Work out the finished part from the listing and answer in its coordinate system (mm). A direction names the side the tool comes from. Round coordinates to 2 decimals unless told otherwise and drop trailing zeros. Write each loop counter-clockwise with the first axis right and the second up, starting at its lowest first coordinate (ties: lowest second). Pieces come first, ordered by that corner, then holes. Notation, with made-up numbers: (3, 21.5) - (28, 21.5) arc R38 ccw to (28, 60.5) - close; hole circle Ø10 at (56, -23.75). An arc over 180 degrees is marked (long way). Answer as a JSON object with one key per item and string values.
Solid Edge part; units mm, degrees
sketch "Sketch1" plane through (0, 0, 0) normal (0, -1, 0) x (1, 0, 0)
  line L0 (0, 32.7794) -> (0, -16.7206)
  line L1 (0, -16.7206) -> (-12, -16.7206)
  line L2 (-12, -16.7206) -> (-12, -42.5202)
  line L3 (-12, -42.5202) -> (39.6634, -42.5202)
  line L4 (39.6634, -42.5202) -> (39.6634, -31.5202)
  line L5 (39.6634, -31.5202) -> (15, -31.5202)
  line L6 (15, -31.5202) -> (15, 8.4798)
  line L7 (15, 8.4798) -> (39.6634, 8.4798)
  line L8 (39.6634, 8.4798) -> (39.6634, 13.9798)
  line L9 (39.6634, 13.9798) -> (23.9789, 13.9798)
  arc A0 (23.9789, 13.9798) -> (15, 22.9587) centre (23.9789, 22.9587) cw
  line L10 (15, 22.9587) -> (15, 32.7794)
  line L11 (15, 32.7794) -> (0, 32.7794)
  circle A1 centre (6, 26.7794) radius 3
  dimension "D1" = 39.6634
  dimension "D2" = 12
  dimension "D3" = 39.6634
extrude "Protrusion1" add sketch "Sketch1" along normal blind 15
sketch "Sketch2" plane through (12.5, -15, -0.5832) normal (0, -1, 0) x (0, 0, 1)
  line L0 (-38.337, 24.5) -> (-38.337, 14.5)
  line L1 (-38.337, 14.5) -> (-41.937, 14.5)
  line L2 (-41.937, 14.5) -> (-41.937, 24.5)
  line L3 (-41.937, 24.5) -> (-38.337, 24.5)
  dimension "D1" = 41.937
  dimension "D2" = 41.937
extrude "Cutout1" cut sketch "Sketch2" against normal through all
sketch "Sketch3" plane through (-6, -7.5, -16.7206) normal (0, 0, 1) x (1, 0, 0)
  line L0 (-1.7229, -2.3191) -> (-0.5, -1.0528)
  line L1 (-0.5, -1.0528) -> (0.7229, -2.3191)
  arc A0 (0.7229, -2.3191) -> (-1.7229, -2.3191) centre (-0.5, -3.5) cw
  line L2 (-1.7229, 4.6809) -> (-0.5, 5.9472)
  line L3 (-0.5, 5.9472) -> (0.7229, 4.6809)
  arc A1 (0.7229, 4.6809) -> (-1.7229, 4.6809) centre (-0.5, 3.5) cw
extrude "Cutout2" cut sketch "Sketch3" against normal through all
sketch "Sketch4" plane through (24.5, -7.5, 13.9798) normal (0, 0, 1) x (1, 0, 0)
  line L0 (8.3834, 1.2545) -> (5.8555, 4.5615)
  line L1 (5.8555, 4.5615) -> (3.3095, 1.2684)
  arc A0 (3.3095, 1.2684) -> (8.3834, 1.2545) centre (5.8411, -0.6889) ccw
extrude "Cutout3" cut sketch "Sketch4" against normal through all
sketch "Sketch5" plane through (15.5, 0, -7.0884) normal (0, 1, 0) x (-1, 0, 0)
  line L0 (-19.7411, -39.4958) -> (-9.7411, -39.4958)
  line L1 (-9.7411, -39.4958) -> (-9.7411, -30.4318)
  line L2 (-9.7411, -30.4318) -> (-19.7411, -30.4318)
  line L3 (-19.7411, -30.4318) -> (-19.7411, -39.4958)
extrude "Cutout4" cut sketch "Sketch5" against normal through all
sketch "Sketch6" plane through (10.293, -7.5, -42.5202) normal (0, 0, -1) x (0, 1, 0)
  line L0 (1.1809, -5.7767) -> (2.4472, -6.9996)
  line L1 (2.4472, -6.9996) -> (1.1809, -8.2225)
  arc A0 (1.1809, -8.2225) -> (1.1809, -5.7767) centre (0, -6.9996) cw
  line L2 (1.1809, 1.926) -> (2.4472, 0.7031)
  line L3 (2.4472, 0.7031) -> (1.1809, -0.5197)
  arc A1 (1.1809, -0.5197) -> (1.1809, 1.926) centre (0, 0.7031) cw
extrude "ExtrudedCutout_5" cut sketch "Sketch6" against normal blind 20
sketch "Sketch7" plane through (0, 0, -33.5884) normal (0, 0, 1) x (1, 0, 0)
  line L0 (8.2462, -7.5) -> (8.2462, 0)
  line L1 (13.7462, 0) -> (8.2462, 0)
  line L2 (13.7462, 0) -> (13.7462, -7.5)
  arc A0 (13.7462, -7.5) -> (8.2462, -7.5) centre (10.9962, -7.5) cw
  line L3 (6.0435, 0) -> (6.0435, -7.5)
  arc A1 (6.0435, -7.5) -> (0.5435, -7.5) centre (3.2935, -7.5) cw
  line L4 (0.5435, -7.5) -> (0.5435, 0)
  line L5 (6.0435, 0) -> (0.5435, 0)
extrude "ExtrudedCutout_8" cut sketch "Sketch7" along normal blind 2.5
properties material "Steel"
Item 1: A cutting plane is placed at C-C (y = -4). Give the number of separate pieces and of enclosed holes in the cut face, and give its area (3 significant figures).
Results found:
{"separate pieces": "4", "enclosed holes": "3", "area": "1,630 mm²"}
Item 2: Each of these flat-tipped pins is pushed along its axis until it touches: P1, Ø5.5, axis at x = 6, z = 26.78, coming from the -Y side; P2, Ø1.5, axis at y = -7, z = -41, coming from the -X side; P3, Ø2.5, axis at x = 11, y = -7.5, coming from the -Z side; P4, Ø3, axis at y = -2.5, z = 1.5, coming from the -X side. Where does it stop, or does it pass through?
Results found:
{"P1": "through", "P2": "x = -2", "P3": "z = -22.52", "P4": "x = 0"}
Item 3: Determine the mould class of faces 1 (the flat face through (0, -7, 8)), 2 (the flat face through (13.746, -4, -32)), 3 (the flat face through (27.9, -5.7, -37.52)) for opening direction Z: pulls with the +Z half, pulls with the -Z half, needs draft (parallel to the pull), parting line crosses it, or undercut.
Results found:
{"face 1": "needs draft", "face 2": "undercut", "face 3": "pulls with the -Z half"}
Item 4: A cutting plane is placed at B-B (x = 19.5). Write down the section's boundary in (y, z).
Results found:
{"outline": "(-15, -42.52) - (0, -42.52) - (0, -31.52) - (-15, -31.52) - close; (-15, 8.48) - (0, 8.48) - (0, 15.18) - (-15, 15.18) - close"}
Item 5: Consider line 1 along X through (y, z) = (-7.5, -26.75); line 2 along X through (y, z) = (-7.5, -39.25); line 3 along X through (y, z) = (-9.25, -34.5). Determine where each line is inside the solid, lowest interval first.
Results found:
{"line 1": "-12 to 1.59, 4.99 to 9.3, 12.7 to 15", "line 2": "-2 to 1.59, 4.99 to 9.3, 12.7 to 25.24, 35.24 to 39.66", "line 3": "-12 to -7.17, -5.83 to 27.32, 33.36 to 39.66"}
Item 6: A cutting plane is placed at D-D (z = 21). Write down the section's boundary in (x, y), and give its area (3 significant figures).
Results found:
{"outline": "(0, -15) - (15.22, -15) - (15.22, 0) - (0, 0) - close", "area": "228 mm²"}
Item 7: For faces 4 (the flat face through (-2, -8, -41)), 5 (the flat face through (25.241, -7, -40)), 6 (the flat face through (29.1, -4.56, 11.27)), determine the directions among +Z, -Z, +X, -X, +Y, -Y from which every point of the face is accessible in a straight line to the end or side of a thin tool.
Results found:
{"face 4": "-Z, -X, +Y, -Y", "face 5": "-Z, +Y, -Y", "face 6": "+Z, -Z"}
Item 8: A cutting plane is placed at A-A (z = -19.5). Write down the section's boundary in (x, y), and give its area (3 significant figures).
Results found:
{"outline": "(-12, -15) - (15, -15) - (15, 0) - (-12, 0) - close; hole (-7.72, -9.82) arc R1.7 ccw (long way) to (-5.28, -9.82) - (-6.5, -8.55) - close; hole (-7.72, -2.82) arc R1.7 ccw (long way) to (-5.28, -2.82) - (-6.5, -1.55) - close", "area": "385 mm²"}
